Verification items for this drawing (mm, ordinates from the low corner). A direction names the side the tool comes from. Coordinates: 2 decimals unless noted, no trailing zeros. Order: outer loops, then holes, each group sorted by start corner. A loop starts at its lowest first (then second) coordinate and runs counter-clockwise, first axis right, second up.
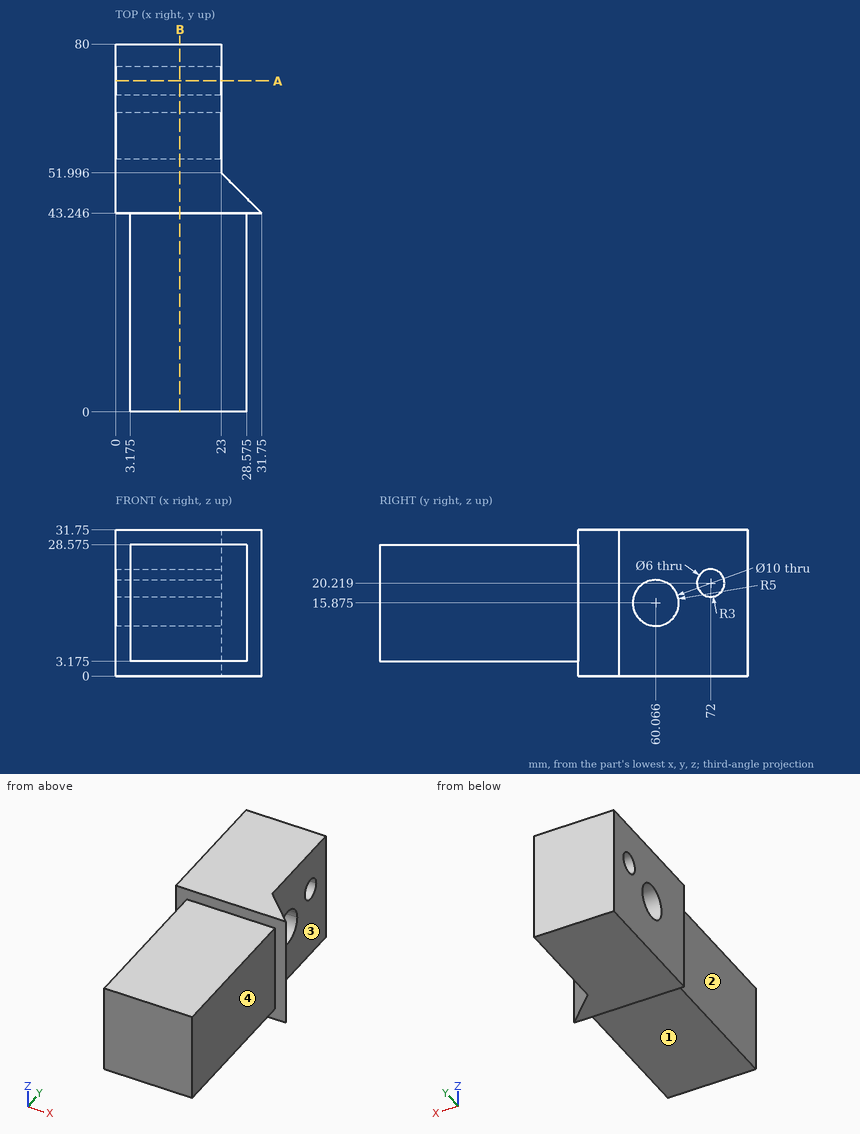
(1) Cross-section at A-A (y = 72). Enter the section's corners in (x, z).
Filled in:
outline: (0, 0) - (23, 0) - (23, 17.22) - (0, 17.22) - close; (0, 23.22) - (23, 23.22) - (23, 31.75) - (0, 31.75) - close
(2) Cross-section at B-B (x = 14). Count the separate pieces of the cut face and the enclosed holes in it, and give its area (3 significant figures).
Filled in:
separate pieces: 1
enclosed holes: 2
area: 2,160 mm2
(3) Thickness scan on probe 1 along Y at (x, z) = (22.5, 20.5) (1 decimal); probe 2 along X at (y, z) = (52.5, 25); probe 3 along Y at (x, z) = (11, 18.5). Record the ranges inside material, lowest first.
Filled in:
probe 1: y = 0 to 58.2, 62 to 69, 75 to 80
probe 2: x = 0 to 23
probe 3: y = 0 to 55.81, 64.32 to 69.54, 74.46 to 80
(4) Go/stop test with flat-tipped pins: P1, Ø10, axis at y = 16, z = 8.5, coming from the +X side (3 decimals); P2, Ø4, axis at x = 15.5, y = 25.5, coming from the +Z side (3 decimals); P3, Ø11.5, axis at y = 60.07, z = 15.87, coming from the +X side. Record where each tip stops, or that it passes through.
Filled in:
P1: stops at x = 28.575
P2: stops at z = 28.575
P3: stops at x = 23
(5) Tool access check on the marked faces 1, 2, 3 and 4. Record the directions out of +Z, -Z, +X, -X, +Y, -Y that give a thin tool (end or side, any length) a straight path to the whole face; none if there is none.
Filled in:
face 1: -Z, +X, -X, -Y
face 2: +Z, -Z, -X, -Y
face 3: +Z, -Z, +X, +Y
face 4: +Z, -Z, +X, -Y
